Part model, mm, in its own coordinate system. Face numbers are marked on the shaded views. A direction names the side the tool comes from. Give positions to 0.01 mm unless a question says otherwise; leave off trailing zeros. Loops run counter-clockwise (first coordinate to the right, second up) from the corner with the lowest first, then second, coordinate; pieces in that order, holes last. Notation, with made-up numbers: (89.25, 28) -> (113.25, 28) arc R12 cw to (113.25, 42) -> close; hole circle Ø4 at (-24.5, 48.25). An arc over 180 degrees is marked (long way). Write item = value, one per line.
from build123d import *

# Parameters (mm, degrees)
F0_R         = 15
F1_DEPTH     = 8.5
F2_T         = -1.35
F4_DEPTH     = 80
F5_R         = 3.5
F6_T3_ANGLE  = 242.5524848973
F6_T9_DEPTH  = 35.6602445691
F6_T13_DEPTH = 35.6602445691


# Not quite as in the source:
# - a fillet or chamfer that OpenCascade refuses, or shapes differently, is made with other operations: its cross-section is extruded or revolved along the edge and cut away or added


with BuildPart() as f1:
    # F0 (on Top) → F1 (new body)
    with BuildSketch(Plane.XY):
        with BuildLine():
            Line((-3.9915498981, -108.0066443023), (3.9915498981, -108.0066443023))
            Line((3.9915498981, -108.0066443023), (3.9915498981, -36.3935431888))
            Line((3.9915498981, -36.3935431888), (19.064122832, -11.5803439591))
            ThreePointArc((19.064122832, -11.5803439591), (0, 22.3057200189), (-19.064122832, -11.5803439591))
            Line((-19.064122832, -11.5803439591), (-3.9915498981, -36.3935431888))
            Line((-3.9915498981, -36.3935431888), (-3.9915498981, -108.0066443023))
        make_face()
        Circle(F0_R, mode=Mode.SUBTRACT)
    extrude(amount=F1_DEPTH)

    # F2
    f2_openings = [f1.faces().sort_by_distance(p)[0] for p in [
        (0, -28.543568, 8.5),
    ]]
    offset(amount=F2_T, openings=f2_openings, kind=Kind.INTERSECTION)

    # F3 (on face) → F4 (cut)
    with BuildSketch(Plane.XZ.offset(108.0066443023)):
        with BuildLine():
            Line((-1.9299790729, 8.5), (-1.9299790729, 5.7166375665))
            ThreePointArc((-1.9299790729, 5.7166375665), (0, 1.5), (1.9299790729, 5.7166375665))
            Line((1.9299790729, 5.7166375665), (1.9299790729, 8.5))
            Line((1.9299790729, 8.5), (-1.9299790729, 8.5))
        make_face()
    extrude(amount=-F4_DEPTH, mode=Mode.SUBTRACT)

    # F5
    f5_edges = [f1.edges().sort_by_distance(p)[0] for p in [
        (3.99155, -36.393543, 4.25),
        (-3.99155, -36.393543, 4.25),
        (-11.527836, -23.986944, 0),
        (3.99155, -72.200094, 0),
        (11.527836, -23.986944, 0),
        (0, 22.30572, 0),
        (-3.99155, -72.200094, 0),
    ]]
    fillet(f5_edges, radius=F5_R)

    # F6: fillet of radius 2.5 on 5 edges, made by hand


with BuildPart() as f6_tool1:
    # F6_s2 → F6_t3 (revolve)
    with BuildSketch(Plane(origin=(0, 0, 0), x_dir=(0, 0, 1), z_dir=(0.519164768, -0.854674174, 0))):
        with BuildLine():
            ThreePointArc((3.85, 20.9557200189), (2.082233047, 20.2234869719), (1.35, 18.4557200189))
            Line((1.35, 18.4557200189), (1.35, 20.9557200189))
            Line((1.35, 20.9557200189), (3.85, 20.9557200189))
        make_face()
    revolve(axis=Axis((0, 0, 1.35), (0, 0, -1)), revolution_arc=F6_T3_ANGLE)


with BuildPart() as f6_tool4:
    # F6_s5 → F6_t6 (revolve)
    with BuildSketch(Plane.XZ):
        with BuildLine():
            ThreePointArc((18.85, 1.35), (17.082233047, 2.082233047), (16.35, 3.85))
            Line((16.35, 3.85), (16.35, 1.35))
            Line((16.35, 1.35), (18.85, 1.35))
        make_face()
    revolve(axis=Axis((0, 0, 1.35), (0, 0, -1)))


with BuildPart() as f6_tool7:
    # F6_s8 → F6_t9 (new body)
    with BuildSketch(Plane(origin=(0, 0, 0), x_dir=(0, 0, 1), z_dir=(0.519164768, -0.854674174, 0))):
        with BuildLine():
            ThreePointArc((3.85, 20.9557200189), (2.082233047, 20.2234869719), (1.35, 18.4557200189))
            Line((1.35, 18.4557200189), (1.35, 20.9557200189))
            Line((1.35, 20.9557200189), (3.85, 20.9557200189))
        make_face()
    extrude(amount=F6_T9_DEPTH)

    split(bisect_by=Plane.YZ.offset(-2.6415498981), keep=Keep.BOTTOM)


with BuildPart() as f6_tool11:
    # F6_s12 → F6_t13 (new body)
    with BuildSketch(Plane(origin=(-18.5135425991, -30.4778900706, 0), x_dir=(0, 0, 1), z_dir=(0.519164768, 0.854674174, 0))):
        with BuildLine():
            ThreePointArc((3.85, 20.9557200189), (2.082233047, 20.2234869719), (1.35, 18.4557200189))
            Line((1.35, 18.4557200189), (1.35, 20.9557200189))
            Line((1.35, 20.9557200189), (3.85, 20.9557200189))
        make_face()
    extrude(amount=F6_T13_DEPTH)

    split(bisect_by=Plane.YZ.offset(2.6415498981), keep=Keep.TOP)


with BuildPart() as f1_1:
    add(f1.part)

    # F6_t15: union F6_tool1, F6_tool4, F6_tool7, F6_tool11
    add([f6_tool1.part, f6_tool4.part, f6_tool7.part, f6_tool11.part])

    # F6_s16 → F6_t17 (revolve, cut)
    with BuildSketch(Plane.XZ):
        with BuildLine():
            ThreePointArc((15, 2.5), (15.732233047, 0.732233047), (17.5, 0))
            Line((17.5, 0), (15, 0))
            Line((15, 0), (15, 2.5))
        make_face()
    revolve(axis=Axis((0, 0, 0), (0, 0, 1)), mode=Mode.SUBTRACT)


solid = f1_1.part
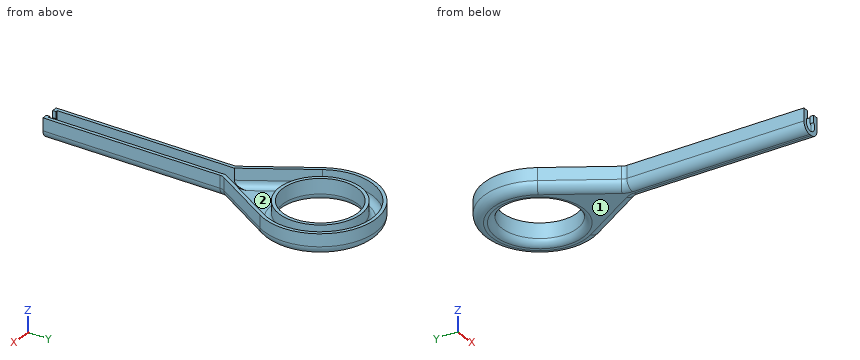
1) Drill centre lines: line 1 along Y through (x, z) = (-0.5, 7.5); line 2 along X through (y, z) = (-69, 7.25); line 3 along Y through (x, z) = (13.5, 4.25). Where is each one in solid material? Low to high. Write a range as [from, to].
Resolved:
line_1 = [-16.34, -14.99], [14.99, 16.34], [20.95, 22.3]
line_2 = [-3.99, -2.64], [2.64, 3.99]
line_3 = [-20.74, -18.14], [-9.22, -6.54], [6.54, 9.22], [16.03, 17.76]
2) Slice it at A-A, the plane z = 7.25. List the corners of the cut face in (x, y), and give its area (3 significant figures).
Resolved:
outline = (-19.06, -11.58) -> (-4.5, -35.56) arc R3.5 cw to (-3.99, -37.37) -> (-3.99, -108.01) -> (-1.93, -108.01) -> (-1.93, -106.66) -> (-2.64, -106.66) -> (-2.64, -36.02) -> (-17.91, -10.88) arc R20.96 cw (long way) to (17.91, -10.88) -> (2.64, -36.02) -> (2.64, -106.66) -> (1.93, -106.66) -> (1.93, -108.01) -> (3.99, -108.01) -> (3.99, -37.37) arc R3.5 cw to (4.5, -35.56) -> (19.06, -11.58) arc R22.31 ccw (long way) to start; circle Ø32.7 at (0, 0); hole circle Ø30 at (0, 0)
area = 531 mm²
3) Slice it at B-B, the plane y = -81. List the corners of the cut face in (x, z), and give its area (3 significant figures).
Resolved:
outline = (-3.99, 3.5) arc R3.5 ccw to (-0.49, 0) -> (0.49, 0) arc R3.5 ccw to (3.99, 3.5) -> (3.99, 8.5) -> (2.64, 8.5) -> (2.64, 1.35) -> (-2.64, 1.35) -> (-2.64, 8.5) -> (-3.99, 8.5) -> close
area = 24.8 mm²
4) Drop flat-ended pins along their axis: P1, Ø1.1, axis at y = -107, z = 7, coming from the -X side; P2, Ø12, axis at x = 14, y = -40, coming from the +Z side; P3, Ø1.5, axis at y = -77.5, z = 6, coming from the +X side; P4, Ø4, axis at x = 0, z = 3, coming from the +Y side. Give the stop position or say it passes through.
Resolved:
P1 = -3.99
P2 = through
P3 = 3.99
P4 = 22.31
5) Which spindle directions (+Z, -Z, +X, -X, +Y, -Y) get a long thin tool onto all of the face, cutting with end or side? Do the marked faces 1 and 2. Say none if no direction does.
Resolved:
face_1 = -Z, +X, -X, +Y, -Y
face_2 = +Z
